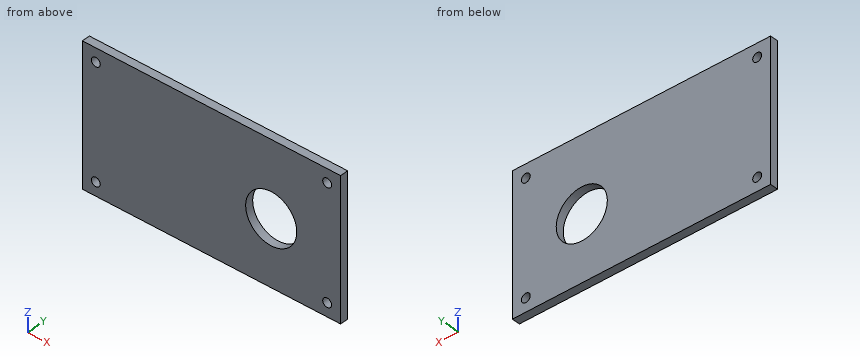
```python
from build123d import *

# Parameters (mm, degrees)
SKETCH1_W           = 96
SKETCH1_H           = 52
BOSS_EXTRUDE1_DEPTH = 3
SKETCH2_R           = 1.65
SKETCH2_R_2         = 9.5
CUT_EXTRUDE1_DEPTH  = 3


with BuildPart() as part:
    # Sketch1 → Boss-Extrude1 (new body)
    with BuildSketch(Plane(origin=(0, 0, 0), x_dir=(1, 0, 0), z_dir=(0, 1, 0))):
        Rectangle(SKETCH1_W, SKETCH1_H)
    extrude(amount=BOSS_EXTRUDE1_DEPTH)

    # Sketch2 → Cut-Extrude1 (cut)
    with BuildSketch(Plane(origin=(0, 3, 0), x_dir=(1, 0, 0), z_dir=(0, 1, 0))):
        with Locations(Location((-43, 21, 0), (0, 0, 270))):
            Circle(SKETCH2_R)
        with Locations(Location((43, 21, 0), (0, 0, 270))):
            Circle(SKETCH2_R)
        with Locations(Location((43, -21, 0), (0, 0, 270))):
            Circle(SKETCH2_R)
        with Locations(Location((-43, -21, 0), (0, 0, 270))):
            Circle(SKETCH2_R)
        with Locations(Location((22.2, 1.8, 0), (0, 0, 270))):
            Circle(SKETCH2_R_2)
    extrude(amount=-CUT_EXTRUDE1_DEPTH, mode=Mode.SUBTRACT)


solid = part.part
```
Work out the finished part from the listing and answer in its coordinate system (mm). Give positions to 0.01 mm unless a question says otherwise; leave off trailing zeros. Loops run counter-clockwise (first coordinate to the right, second up) from the corner with the lowest first, then second, coordinate; pieces in that order, holes last. Notation, with made-up numbers: (64.25, 62) -> (72.25, 62) arc R9 cw to (72.25, 66) -> close; hole circle Ø1 at (47, 54). An arc over 180 degrees is marked (long way). Put each result on its own line as item: value. Start each with the question number.
Item 1: The part is cut by section B-B (z = 21). Give the vertices of the cut face in (x, y).
Item 2: Find the intervals of material crossed by L1, parallel to X at y = 2.4, z = 21; L2, parallel to X at y = 0.7, z = -1.8; L3, parallel to X at y = 0.4, z = -3.5, in increasing order. Write a range as [from, to].
Item 3: Each of these flat-tipped pins is pushed along its axis until it touches: P1, Ø24.5, axis at x = 22.2, z = -1.8, coming from the -Y side; P2, Ø2.5, axis at x = -43, z = -21, coming from the -Y side. Where does it stop, or does it pass through?
Item 4: The part is cut by section D-D (x = 43). Give the vertices of the cut face in (y, z).
Item 5: The part is cut by section C-C (y = 0.6). Give the vertices of the cut face in (x, z).
Item 6: The part is cut by section A-A (x = 22.2). Give the vertices of the cut face in (y, z).
Answers below:
1. outline: (-48, 0) -> (-44.65, 0) -> (-44.65, 3) -> (-48, 3) -> close; (-41.35, 0) -> (41.35, 0) -> (41.35, 3) -> (-41.35, 3) -> close; (44.65, 0) -> (48, 0) -> (48, 3) -> (44.65, 3) -> close
2. L1: [-48, -44.65], [-41.35, 41.35], [44.65, 48]
2. L2: [-48, 12.7], [31.7, 48]
2. L3: [-48, 12.85], [31.55, 48]
3. P1: y = 0
3. P2: through
4. outline: (0, -26) -> (3, -26) -> (3, -22.65) -> (0, -22.65) -> close; (0, -19.35) -> (3, -19.35) -> (3, 19.35) -> (0, 19.35) -> close; (0, 22.65) -> (3, 22.65) -> (3, 26) -> (0, 26) -> close
5. outline: (-48, -26) -> (48, -26) -> (48, 26) -> (-48, 26) -> close; hole circle Ø3.3 at (-43, -21); hole circle Ø3.3 at (-43, 21); hole circle Ø19 at (22.2, -1.8); hole circle Ø3.3 at (43, -21); hole circle Ø3.3 at (43, 21)
6. outline: (0, -26) -> (3, -26) -> (3, -11.3) -> (0, -11.3) -> close; (0, 7.7) -> (3, 7.7) -> (3, 26) -> (0, 26) -> close
